from build123d import *

# Parameters (mm, degrees)
SKETCH_1_R      = 22.65
EXTRUDE_1_DEPTH = 2


with BuildPart() as part:
    # 草图1 → 凸台-拉伸1 (new body)
    with BuildSketch(Plane(origin=(0, 0, 0), x_dir=(1, 0, 0), z_dir=(0, 1, 0))):
        with BuildLine():
            Line((0, -77.7), (46.435, -77.7))
            Line((46.435, -77.7), (53.35, -63.178332735))
            ThreePointArc((53.35, -63.178332735), (62.85, -57.18), (72.35, -63.178332735))
            Line((72.35, -63.178332735), (79.265, -77.7))
            Line((79.265, -77.7), (125.7, -77.7))
            Line((125.7, -77.7), (125.7, 0))
            Line((125.7, 0), (0, 0))
            Line((0, 0), (0, -77.7))
        make_face()
        with Locations(Location((32.16, -38.85, 0), (0, 0, 270))):
            Circle(SKETCH_1_R, mode=Mode.SUBTRACT)
        with Locations(Location((93.54, -38.85, 0), (0, 0, 270))):
            Circle(SKETCH_1_R, mode=Mode.SUBTRACT)
    extrude(amount=EXTRUDE_1_DEPTH)


solid = part.part
Work out the finished part from the listing and answer in its coordinate system (mm). A direction names the side the tool comes from. Coordinates: 2 decimals unless noted, no trailing zeros. Write each loop counter-clockwise with the first axis right and the second up, starting at its lowest first coordinate (ties: lowest second). Pieces come first, ordered by that corner, then holes.
1. The part is cut by section B-B, the plane z = 27. Write down the section's boundary in (x, y).
Results list:
outline: (0, 0) - (12.86, 0) - (12.86, 2) - (0, 2) - close; (51.46, 0) - (74.24, 0) - (74.24, 2) - (51.46, 2) - close; (112.84, 0) - (125.7, 0) - (125.7, 2) - (112.84, 2) - close
2. For a pull along X with two mould halves and no side action, classify faces 1 (the flat face through (75.76, 0.99, 70.34)), 2 (the flat face through (62, 2, 38)) as +X half, -X half, draft (parallel to the pull), parting line (faces both ways), or undercut.
Results list:
face 1: undercut
face 2: draft
3. The part is cut by section A-A, the plane x = 32.16. Write down the section's boundary in (y, z).
Results list:
outline: (0, 0) - (2, 0) - (2, 16.2) - (0, 16.2) - close; (0, 61.5) - (2, 61.5) - (2, 77.7) - (0, 77.7) - close
4. The part is cut by section C-C, the plane y = 0.7. Write down the section's boundary in (x, z) (3 decimals), and give its area (3 significant figures).
Results list:
outline: (0, 0) - (125.7, 0) - (125.7, 77.7) - (79.265, 77.7) - (72.35, 63.178) arc R10.522 cw to (53.35, 63.178) - (46.435, 77.7) - (0, 77.7) - close; hole circle Ø45.3 at (32.16, 38.85); hole circle Ø45.3 at (93.54, 38.85)
area: 6,090 mm2
5. For faces 3 (the flat face through (49.844, 0.986, 70.541)), 4 (the flat face through (62, 0, 38)), determine the directions among +Z, -Z, +X, -X, +Y, -Y from which every point of the face is accessible in a straight line to the end or side of a thin tool.
Results list:
face 3: +Z, +Y, -Y
face 4: +Z, -Z, +X, -X, -Y
6. The part is cut by section D-D, the plane z = 38.85. Write down the section's boundary in (x, y).
Results list:
outline: (0, 0) - (9.51, 0) - (9.51, 2) - (0, 2) - close; (54.81, 0) - (70.89, 0) - (70.89, 2) - (54.81, 2) - close; (116.19, 0) - (125.7, 0) - (125.7, 2) - (116.19, 2) - close
7. Consider line 1 along X through (y, z) = (0.85, 38.85); line 2 along Z through (x, y) = (15, 1.2); line 3 along X through (y, z) = (0.25, 48). Determine where each line is inside the solid, lowest interval first.
Results list:
line 1: x = 0 to 9.51, 54.81 to 70.89, 116.19 to 125.7
line 2: z = 0 to 24.07, 53.63 to 77.7
line 3: x = 0 to 11.44, 52.88 to 72.82, 114.26 to 125.7
